Source: CAD feature listing. Evaluate the final solid. Frame: model axes, mm. A direction names the side the tool comes from. Round coordinates to 2 decimals unless told otherwise and drop trailing zeros. Loops run counter-clockwise (first coordinate to the right, second up) from the corner with the lowest first, then second, coordinate; pieces in that order, holes last.
Item 1: Ray query, L1, parallel to Z at x = -1.8, y = 0; L2, parallel to X at y = -1, z = 2; L3, parallel to Y at x = -1.4, z = 42. Return the intervals inside material, ascending.
Item 2: Section query A-A on y = 0. Return loops of the section in (x, z), then the cut area to 3 significant figures.
Item 3: Access query for faces 1 (the flat face through (0.9, 1.4, 3)), 2 (the flat face through (-0.9, 1.4, 43)), 3 (the flat face through (2, 0, 23)). Directions: +Z, -Z, +X, -X, +Y, -Y. A direction counts if a zero-diameter tool reaches every point of the face in a straight line with its end or side. Return the directions, or none.
Item 4: Section query C-C on z = 7.5. Return loops of the section in (x, y), then the cut area to 3 significant figures.
```python
from build123d import *

# Parameters (mm, degrees)
CROQUIS1_R              = 1.5
SALIENTE_EXTRUIR1_DEPTH = 46
SALIENTE_EXTRUIR2_DEPTH = 43
CORTAR_EXTRUIR1_START   = -3
CROQUIS3_R              = 3.153795035
CROQUIS3_R_2            = 1.5
CORTAR_EXTRUIR1_DEPTH   = 3


with BuildPart() as part:
    # Croquis1 → Saliente-Extruir1 (new body)
    with BuildSketch(Plane.XY):
        Circle(CROQUIS1_R)
    extrude(amount=SALIENTE_EXTRUIR1_DEPTH)

    # Croquis2 → Saliente-Extruir2 (add)
    with BuildSketch(Plane.XY.offset(46)):
        Polygon((-0.828427125, -2), (0.828427125, -2), (2, -0.828427125), (2, 0.828427125), (0.828427125, 2), (-0.828427125, 2), (-2, 0.828427125), (-2, -0.828427125), align=None)
    extrude(amount=-SALIENTE_EXTRUIR2_DEPTH)

    # Croquis3 → Cortar-Extruir1 (cut)
    with BuildSketch(Plane.XY.offset(46).offset(CORTAR_EXTRUIR1_START)):
        Circle(CROQUIS3_R)
        with Locations(Location((0, 0, 0), (0, 0, 180))):
            Circle(CROQUIS3_R_2, mode=Mode.SUBTRACT)
    extrude(amount=CORTAR_EXTRUIR1_DEPTH, mode=Mode.SUBTRACT)


solid = part.part
```
Data:
1. L1: z = 3 to 43
1. L2: x = -1.12 to 1.12
1. L3: y = -1.43 to 1.43
2. outline: (-2, 3) - (-1.5, 3) - (-1.5, 0) - (1.5, 0) - (1.5, 3) - (2, 3) - (2, 43) - (1.5, 43) - (1.5, 46) - (-1.5, 46) - (-1.5, 43) - (-2, 43) - close
2. area: 178 mm2
3. face 1: -Z
3. face 2: +Z
3. face 3: +Z, -Z, +X, +Y, -Y
4. outline: (-2, -0.83) - (-0.83, -2) - (0.83, -2) - (2, -0.83) - (2, 0.83) - (0.83, 2) - (-0.83, 2) - (-2, 0.83) - close
4. area: 13.3 mm2
